Check sheet for the drawn part. Datum: minimum x, y, z corner. Units: mm. A direction names the side the tool comes from. Coordinates: 2 decimals unless noted, no trailing zeros. Order: outer loops, then holes, each group sorted by start corner. A loop starts at its lowest first (then second) coordinate and runs counter-clockwise, first axis right, second up. Notation, with made-up numbers: (4, -36) - (33, -36) arc R30 ccw to (33, 0) - close; hole circle Ø2 at (-1, 17.25). An arc over 180 degrees is marked (long way). One line per item, written item: value. Start each with the question number.
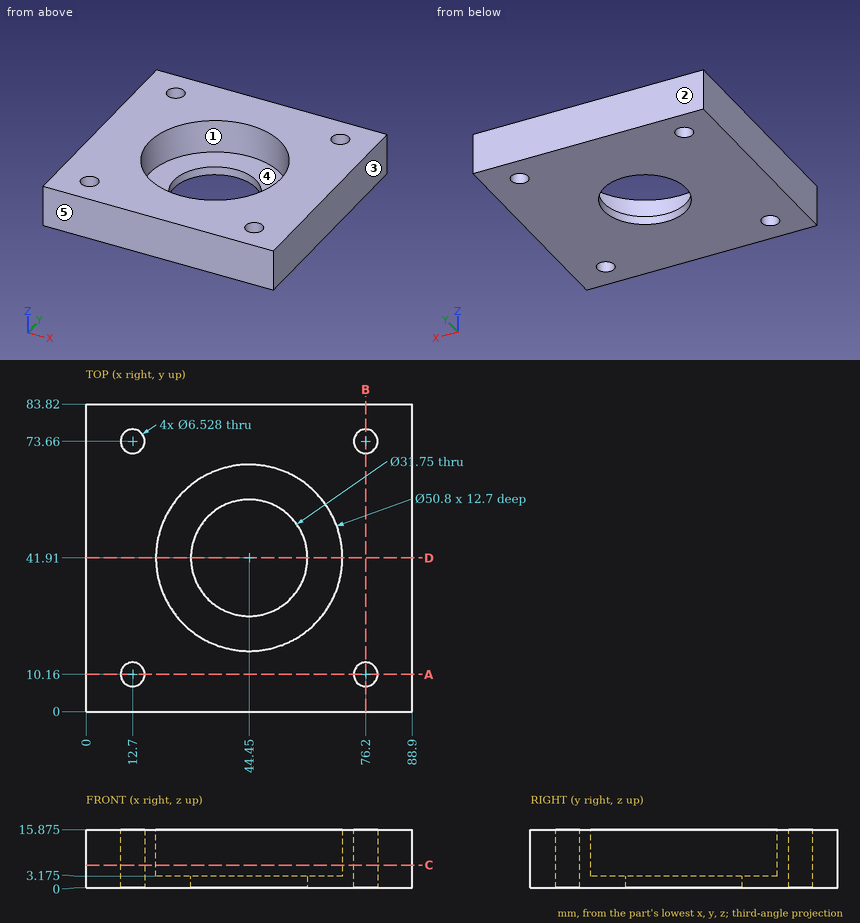
Q1. Set-up check for the marked faces 4 and 5: record each of +Z, -Z, +X, -X, +Y, -Y from which the full face is reachable in a straight line by a thin tool's end or side.
Q2. Cross-section at D-D, the plane y = 41.91. Enter the section's corners in (x, z) (3 decimals).
Q3. Material ranges on probe 1 along X at (y, z) = (74, 8); probe 2 along Y at (x, z) = (12.7, 5.5); probe 3 along Y at (x, z) = (73.5, 2.5) (1 decimal), recorded low to high.
Q4. Cross-section at A-A, the plane y = 10.16. Enter the section's corners in (x, z) (1 decimal), and give its area (3 significant figures).
Q5. Gauge pin test, flat end, axial feed: P1, Ø8, axis at x = 53, y = 52.5, coming from the +Z side (3 decimals). Record the tip position at first contact, or that the pin passes through.
Q6. Cross-section at B-B, the plane x = 76.2. Enter the section's corners in (y, z) (1 decimal).
Q7. Release check for a two-part mould opening along Y. For the marked faces 1, 2 and 3 record: released by +Y, released by -Y, zero draft, split by the parting line, or undercut.
Q8. Cross-section at C-C, the plane z = 6.25. Enter the section's corners in (x, y), and give its area (3 significant figures).
Check result:
1. face 4: +Z
1. face 5: +Z, -Z, +X, -X, -Y
2. outline: (0, 0) - (28.575, 0) - (28.575, 3.175) - (19.05, 3.175) - (19.05, 15.875) - (0, 15.875) - close; (60.325, 0) - (88.9, 0) - (88.9, 15.875) - (69.85, 15.875) - (69.85, 3.175) - (60.325, 3.175) - close
3. probe 1: x = 0 to 9.45, 15.95 to 72.95, 79.45 to 88.9
3. probe 2: y = 0 to 6.9, 13.42 to 70.4, 76.92 to 83.82
3. probe 3: y = 0 to 8.3, 12 to 71.8, 75.5 to 83.8
4. outline: (0, 0) - (9.4, 0) - (9.4, 15.9) - (0, 15.9) - close; (16, 0) - (72.9, 0) - (72.9, 15.9) - (16, 15.9) - close; (79.5, 0) - (88.9, 0) - (88.9, 15.9) - (79.5, 15.9) - close
4. area: 1,200 mm2
5. P1: stops at z = 3.175
6. outline: (0, 0) - (6.9, 0) - (6.9, 15.9) - (0, 15.9) - close; (13.4, 0) - (70.4, 0) - (70.4, 15.9) - (13.4, 15.9) - close; (76.9, 0) - (83.8, 0) - (83.8, 15.9) - (76.9, 15.9) - close
7. face 1: undercut
7. face 2: released by +Y
7. face 3: zero draft
8. outline: (0, 0) - (88.9, 0) - (88.9, 83.82) - (0, 83.82) - close; hole circle Ø6.53 at (12.7, 10.16); hole circle Ø6.53 at (12.7, 73.66); hole circle Ø50.8 at (44.45, 41.91); hole circle Ø6.53 at (76.2, 10.16); hole circle Ø6.53 at (76.2, 73.66)
8. area: 5,290 mm2
